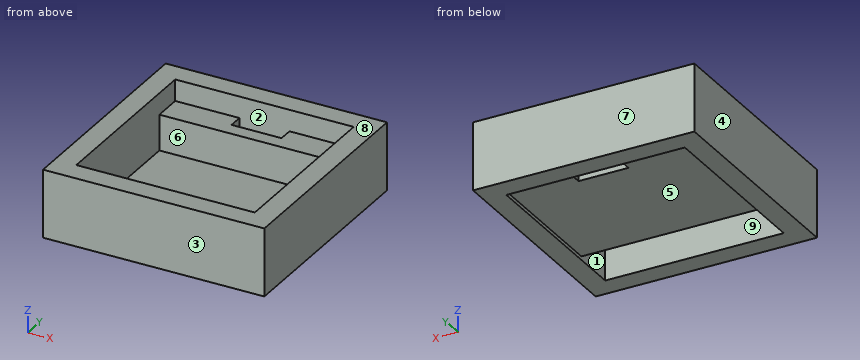
from build123d import *

# Parameters (mm, degrees)
F0_W     = 310
F0_H     = 310
F0_W_2   = 250
F0_H_2   = 250
F1_DEPTH = 90
F3_DEPTH = 60
F4_W     = 250
F4_H     = 140
F4_H_2   = 10
F5_DEPTH = 10
F6_DEPTH = 30
F7_DEPTH = 5


with BuildPart() as f1:
    # F0 (on Top) → F1 (new body)
    with BuildSketch(Plane.XY):
        Rectangle(F0_W, F0_H)
        Rectangle(F0_W_2, F0_H_2, mode=Mode.SUBTRACT)
    extrude(amount=F1_DEPTH)

    # F2 (on face) → F3 (join)
    with BuildSketch(Plane(origin=(0, 0, 0), x_dir=(1, 0, 0), z_dir=(0, 0, -1))):
        Polygon((-125, -85), (-125, -125), (-35, -125), (-35, -105), (35, -105), (35, -125), (125, -125), (125, -85), align=None)
    extrude(amount=-F3_DEPTH)

    # F4 (on face) → F5 (join)
    with BuildSketch(Plane(origin=(0, 0, 0), x_dir=(1, 0, 0), z_dir=(0, 0, -1))):
        with Locations((0, -15)):
            Rectangle(F4_W, F4_H)
        with Locations((0, 60)):
            Rectangle(F4_W, F4_H_2)
    extrude(amount=-F5_DEPTH)

    # F4 (on face) → F6 (join)
    with BuildSketch(Plane(origin=(0, 0, 0), x_dir=(1, 0, 0), z_dir=(0, 0, -1))):
        with Locations((0, 60)):
            Rectangle(F4_W, F4_H_2)
    extrude(amount=-F6_DEPTH)

    # F0 (on Top) → F7 (join)
    with BuildSketch(Plane.XY):
        Rectangle(F0_W, F0_H)
        Rectangle(F0_W_2, F0_H_2, mode=Mode.SUBTRACT)
    extrude(amount=-F7_DEPTH)


solid = f1.part
Can you work these out from the model? Positions are in its coordinate system, mm. Face numbers are marked on the shaded views. A direction names the side the tool comes from. Give positions to 0.01 mm unless a question says otherwise; leave off trailing zeros. Loops run counter-clockwise (first coordinate to the right, second up) from the corner with the lowest first, then second, coordinate; pieces in that order, holes last. Notation, with made-up numbers: (16.25, -39.5) - (66.25, -39.5) arc R28 cw to (66.25, -3.5) - close; hole circle Ø10 at (-35.75, 18). An arc over 180 degrees is marked (long way). Answer as a JSON object with one key per item and string values.
Q1. Will these pins go through, and if not, where does the flat tip stop? P1, Ø1, axis at x = 6.5, y = 48, coming from the +Z side; P2, Ø3, axis at x = -102.5, y = 78, coming from the -Z side; P3, Ø8, axis at x = 46.5, y = -59, coming from the +Z side.
Geometry says:
{"P1": "z = 10", "P2": "z = 0", "P3": "z = 30"}
Q2. Imagine slicing it at A-A on y = -113.5. Write out the boundary of the cut face in (x, z).
Geometry says:
{"outline": "(-155, -5) - (-125, -5) - (-125, 90) - (-155, 90) - close; (125, -5) - (155, -5) - (155, 90) - (125, 90) - close"}
Q3. Which directions (+Z, -Z, +X, -X, +Y, -Y) give clear straight access to the entire face, cutting with the end or side of a thin tool? Please do the marked faces 5, 6, 7, 8 and 9.
Geometry says:
{"face 5": "-Z", "face 6": "+Z", "face 7": "+Z, -Z, +X, -X, +Y", "face 8": "+Z, +X, -X, +Y, -Y", "face 9": "+Z, -Z"}
Q4. If we mould it in two halves opening along X, with no side actions, what happens to the marked faces 1, 2, 3 and 4? For each: pulls with the +X half, pulls with the -X half, needs draft (parallel to the pull), parting line crosses it, or undercut.
Geometry says:
{"face 1": "undercut", "face 2": "undercut", "face 3": "needs draft", "face 4": "pulls with the -X half"}
Q5. Imagine slicing it at C-C on x = -7. Write out the boundary of the cut face in (y, z).
Geometry says:
{"outline": "(-155, -5) - (-125, -5) - (-125, 90) - (-155, 90) - close; (-65, 0) - (105, 0) - (105, 60) - (85, 60) - (85, 10) - (-55, 10) - (-55, 30) - (-65, 30) - close; (125, -5) - (155, -5) - (155, 90) - (125, 90) - close"}
Q6. Imagine slicing it at D-D on z = 19. Write out the boundary of the cut face in (x, y).
Geometry says:
{"outline": "(-155, -155) - (155, -155) - (155, 155) - (-155, 155) - close; hole (-125, -125) - (125, -125) - (125, -65) - (-125, -65) - close; hole (-125, -55) - (125, -55) - (125, 85) - (-125, 85) - close; hole (-35, 105) - (35, 105) - (35, 125) - (-35, 125) - close"}
Q7. If I drill on L1, parallel to Y at x = -79.5, z = 28.5; L2, parallel to X at y = 104, z = 68; L3, parallel to Y at x = 74.5, z = 9, over which ranges is the centre line in solid material (lowest first)?
Geometry says:
{"L1": "-155 to -125, -65 to -55, 85 to 155", "L2": "-155 to -125, 125 to 155", "L3": "-155 to -125, -65 to 155"}
Q8. Imagine slicing it at B-B on z = 44. Write out the boundary of the cut face in (x, y), plus the area to 3 significant figures.
Geometry says:
{"outline": "(-155, -155) - (155, -155) - (155, 155) - (-155, 155) - close; hole (-125, -125) - (125, -125) - (125, 85) - (-125, 85) - close; hole (-35, 105) - (35, 105) - (35, 125) - (-35, 125) - close", "area": "42,200 mm²"}
